Design review of the part built by this model. Coordinates are the model's own, in mm. A direction names the side the tool comes from. Round coordinates to 2 decimals unless told otherwise and drop trailing zeros. Write each loop counter-clockwise with the first axis right and the second up, starting at its lowest first coordinate (ties: lowest second). Pieces come first, ordered by that corner, then holes. Notation, with made-up numbers: (-5, 34) -> (25, 34) arc R29 ccw to (25, 68) -> close; hole circle Ø10 at (13, -28.5). An arc over 180 degrees is marked (long way). One line per question, with ' | ' between items. Start each with the question number.
1) Consider section D-D (x = 19). Give the boundary of the cut face in (y, z).
2) Mouldability with a two-part tool opening along Z and no side actions: class faces 4 (the flat face through (-1, 1, -30)), 5 (the cylindrical face through (19.71, 10.48, -25.61)), 6 (the flat face through (45, 1, 0)) as +Z half, -Z half, draft (parallel to the pull), parting line (faces both ways), or undercut.
3) For faces 1 (the cylindrical face through (-37.66, 5.45, -26.61)), 2 (the flat face through (-22.054, 1, 0)), 3 (the flat face through (-39, 12, 24)), list the 3-axis set-ups (+Z, -Z, +X, -X, +Y, -Y) from which the entire face can be reached by the end or side of a thin tool; tool diameter is ignored.
4) Insertion check: pin 1 Ø12 at (x, z) = (-30.5, 12.5) entering from +Y. The pin has a flat end and moves straight along its axis. Give the tip position at first contact, or say it passes through.
5) Consider section B-B (z = 6.5). Give the boundary of the cut face in (x, y).
6) For probe 1 along X at (y, z) = (9.5, -24.5); probe 2 along Z at (x, y) = (6, 1); probe 3 along Y at (x, z) = (-37, 21), list the stretches that pass through material, from the lowest coordinate up.
7) Consider section A-A (x = 9). Give the boundary of the cut face in (y, z).
8) Consider section C-C (y = 3). Give the boundary of the cut face in (x, z), then the cut area to 3 significant figures.
```python
from build123d import *

# Parameters (mm, degrees)
CROQUIS1_W              = 90
CROQUIS1_H              = 60
SALIENTE_EXTRUIR1_DEPTH = 2
CROQUIS2_R              = 2.5
SALIENTE_EXTRUIR2_DEPTH = 7
CROQUIS3_R              = 0.98725552
CROQUIS3_R_2            = 1.31678764
CROQUIS3_R_3            = 1.399541148
CROQUIS3_R_4            = 1.294656753
SALIENTE_EXTRUIR3_DEPTH = 3
CROQUIS4_W              = 35.666485166
CROQUIS4_H              = 22.011405482
CORTAR_EXTRUIR1_DEPTH   = 3


with BuildPart() as part:
    # Croquis1 → Saliente-Extruir1 (new body)
    with BuildSketch(Plane(origin=(0, 0, 0), x_dir=(1, 0, 0), z_dir=(0, 1, 0))):
        Rectangle(CROQUIS1_W, CROQUIS1_H)
    extrude(amount=SALIENTE_EXTRUIR1_DEPTH)

    # Croquis2 → Saliente-Extruir2 (add)
    with BuildSketch(Plane(origin=(0, 2, 0), x_dir=(1, 0, 0), z_dir=(0, 1, 0))):
        with Locations((-39, 24.5)):
            Circle(CROQUIS2_R)
        with Locations((19, 24.5)):
            Circle(CROQUIS2_R)
        with Locations((19, -24.5)):
            Circle(CROQUIS2_R)
        with Locations((-39, -24.5)):
            Circle(CROQUIS2_R)
    extrude(amount=SALIENTE_EXTRUIR2_DEPTH)

    # Croquis3 → Saliente-Extruir3 (add)
    with BuildSketch(Plane(origin=(0, 9, 0), x_dir=(1, 0, 0), z_dir=(0, 1, 0))):
        with Locations((-39, 24.5)):
            Circle(CROQUIS3_R)
        with Locations((19, 24.5)):
            Circle(CROQUIS3_R_2)
        with Locations((19, -24.5)):
            Circle(CROQUIS3_R_3)
        with Locations((-39, -24.5)):
            Circle(CROQUIS3_R_4)
    extrude(amount=SALIENTE_EXTRUIR3_DEPTH)

    # Croquis4 → Cortar-Extruir1 (cut)
    with BuildSketch(Plane(origin=(0, 2, 0), x_dir=(1, 0, 0), z_dir=(0, 1, 0))):
        with Locations((-4.220482568, 0)):
            Rectangle(CROQUIS4_W, CROQUIS4_H)
    extrude(amount=-CORTAR_EXTRUIR1_DEPTH, mode=Mode.SUBTRACT)


solid = part.part
```
From the geometry:
1) outline: (0, -30) -> (2, -30) -> (2, -27) -> (9, -27) -> (9, -25.82) -> (12, -25.82) -> (12, -23.18) -> (9, -23.18) -> (9, -22) -> (2, -22) -> (2, 22) -> (9, 22) -> (9, 23.1) -> (12, 23.1) -> (12, 25.9) -> (9, 25.9) -> (9, 27) -> (2, 27) -> (2, 30) -> (0, 30) -> close
2) face 4: -Z half | face 5: undercut | face 6: draft
3) face 1: +Y | face 2: +Y, -Y | face 3: +Z, -Z, +X, -X, +Y
4) pin 1: stops at y = 2
5) outline: (-45, 0) -> (-22.05, 0) -> (-22.05, 2) -> (-45, 2) -> close; (13.61, 0) -> (45, 0) -> (45, 2) -> (13.61, 2) -> close
6) probe 1: x = -39.99 to -38.01, 17.68 to 20.32 | probe 2: z = -30 to -11.01, 11.01 to 30 | probe 3: y = 0 to 2
7) outline: (0, -30) -> (2, -30) -> (2, -11.01) -> (0, -11.01) -> close; (0, 11.01) -> (2, 11.01) -> (2, 30) -> (0, 30) -> close
8) outline: circle Ø5 at (-39, -24.5); circle Ø5 at (-39, 24.5); circle Ø5 at (19, -24.5); circle Ø5 at (19, 24.5) | area: 78.5 mm2
